Source: CAD feature listing. Evaluate the final solid. Frame: model axes, mm. A direction names the side the tool comes from. Round coordinates to 2 decimals unless told otherwise and drop trailing zeros. Write each loop counter-clockwise with the first axis right and the second up, starting at its lowest first coordinate (ties: lowest second). Pieces come first, ordered by that corner, then holes. Notation, with made-up numbers: (65.25, 87) - (105.25, 87) arc R16 cw to (105.25, 100) - close; hole circle Ø10 at (51.5, 50.25). An arc over 180 degrees is marked (long way). Write item = value, one per line. Start each with the question number.
```python
from build123d import *

# Parameters (mm, degrees)
SKETCH3_R          = 3
CUT_EXTRUDE1_DEPTH = 24


with BuildPart() as part:
    # Sketch2 → Revolve1 (revolve)
    with BuildSketch(Plane.XY):
        Polygon((0, 5.73931272), (68, 5.73931272), (68, 35.73931272), (66, 35.73931272), (62.360297657, 25.73931272), (58.993760511, 25.73931272), (55.975766288, 34.031183701), (53.975766288, 34.031183701), (53.975766288, 26.307716676), (51.619965111, 26.307716676), (49.229261585, 19.73931272), (43.229261585, 19.73931272), (39.953529476, 28.73931272), (37.953529476, 28.73931272), (37.953529476, 19.662434754), (34.588066023, 19.662434754), (32.432225909, 13.73931272), (29.593231819, 13.73931272), (25.953529476, 23.73931272), (23.953529476, 23.73931272), (23.953529476, 21.23931272), (22.901415474, 21.23931272), (18.897742897, 10.23931272), (15.914444309, 10.23931272), (12.820697317, 18.73931272), (12, 18.73931272), (12, 16.23931272), (0, 16.23931272), align=None)
    revolve(axis=Axis((0, 1.23931272, 0), (-1, 0, 0)))

    # Sketch3 → Cut-Extrude1 (cut)
    with BuildSketch(Plane(origin=(0, 0, 0), x_dir=(1, 0, 0), z_dir=(0, 1, 0))):
        with Locations(Location((6, 0, 0), (0, 0, 180))):
            Circle(SKETCH3_R)
    extrude(amount=CUT_EXTRUDE1_DEPTH, mode=Mode.SUBTRACT)


solid = part.part
```
(1) Contact query for flat-ended pins moving along their axis: P1, Ø1, axis at y = -14, z = 22, coming from the -X side; P2, Ø8, axis at x = 9.5, y = 24.5, coming from the +Z side; P3, Ø8, axis at x = 6, z = 0, coming from the +Y side; P4, Ø3, axis at x = 8.5, z = 15, coming from the +Y side. Output: stop coordinate, or through.
(2) Section A-A (z = 0). Count the separate pieces of the cut face and the enclosed holes in it, plus the area to 3 significant figures.
(3) Ray query, L1, parallel to X at y = 13.5, z = 0; L2, parallel to X at y = -8.5, z = -11.5; L3, parallel to Y at x = 37, z = 0. Return the intervals inside material, ascending. Write a range as from..to.
(4) Pull-direction query (Z, two-part tool) for faces 4 (the cylindrical face through (12.405, -12.648, 10.648)), 5 (the flat face through (53.976, -6.2, 24.1)), 6 (the cylindrical face through (3.14, 10.33, 0.9)); classes: +Z half, -Z half, draft (parallel to the pull), parting line (faces both ways), or undercut.
(5) Reachability of faces 1 (the cylindrical face through (54.962, 32.517, -9.85)), 2 (the flat face through (68, -6, 0)), 3 (the cylindrical face through (30.993, 13.162, -3.755)) from +Z, -Z, +X, -X, +Y, -Y: full face, straight path, thin tool, end or side. Return the list, or none.
(6) Section B-B (x = 55). Return the cut outline in (y, z).
(7) Section C-C (x = 6). Return the cut outline in (y, z), plus the area to 3 significant figures.
(8) Section D-D (x = 31). Return the cut outline in (y, z), plus the area to 3 significant figures.
Solution:
q1.P1 = 37.95
q1.P2 = through
q1.P3 = 16.24
q1.P4 = 7.78
q2.separate_pieces = 3
q2.enclosed_holes = 0
q2.area = 2,010 mm^2
q3.L1 = 0..3, 9..14.73, 20.08..68
q3.L2 = 12..13.71, 21.11..28.66, 33.37..68
q3.L3 = -17.18..-3.26, 5.74..19.66
q4.face_4 = parting line
q4.face_5 = draft
q4.face_6 = undercut
q5.face_1 = -X
q5.face_2 = +Z, -Z, +X, +Y, -Y
q5.face_3 = none
q6.outline = circle Ø65.58 at (1.24, 0); hole circle Ø9 at (1.24, 0)
q7.outline = (4.59, -3) arc R4.5 cw (long way) to (4.59, 3) - (15.94, 3) arc R15 ccw (long way) to (15.94, -3) - close
q7.area = 579 mm^2
q8.outline = circle Ø25 at (1.24, 0); hole circle Ø9 at (1.24, 0)
q8.area = 427 mm^2
